Geometry check sheet. Reference: the model listing, model coordinates, mm. Round coordinates to 2 decimals unless told otherwise and drop trailing zeros. Order: outer loops, then holes, each group sorted by start corner. A loop starts at its lowest first (then second) coordinate and runs counter-clockwise, first axis right, second up.
(1) Go/stop test with flat-tipped pins: pin 1 (4 mm diameter, centred on y = 22.5, z = 2.5, fed in from +X); pin 2 (3 mm diameter, centred on x = 10.5, z = 5, fed in from -Y). Record where each tip stops, or that it passes through.
(2) Material ranges on line 1 along Y through (x, z) = (0, 2.95); line 2 along X through (y, z) = (15.5, 6); line 3 along Y through (x, z) = (8.5, 2), recorded low to high.
(3) Sectioned sample at A-A (x = 0). Record the boundary of the cut face in (y, z), plus the area to 3 significant figures.
(4) Release check for a two-part mould opening along Y. For faces 1 (the face through (-8.67, -39.05, 3.48)), 2 (the face through (-1, -8, 0)), 3 (the face through (5.97, 20.36, 3.47)) record: +Y half, -Y half, draft (parallel to the pull), parting line (faces both ways), or undercut.
(5) Sectioned sample at B-B (z = 3.75). Record the boundary of the cut face in (x, y), plus the area to 3 significant figures.
from build123d import *

# Parameters (mm, degrees)
F0_R     = 40
F0_R_2   = 11.1
F1_DEPTH = 7
F2_SIZE  = 2
F3_SIZE2 = 1.5
F3_SIZE  = 0.5


with BuildPart() as f1:
    # F0 (on Top) → F1 (new body)
    with BuildSketch(Plane.XY):
        Circle(F0_R)
        with Locations((0, 11)):
            Circle(F0_R_2, mode=Mode.SUBTRACT)
    extrude(amount=F1_DEPTH)

    # F2
    f2_edges = [f1.edges().sort_by_distance(p)[0] for p in [
        (-40, 0, 7),
        (-40, 0, 0),
    ]]
    chamfer(f2_edges, length=F2_SIZE)

    # F3
    f3_edges = [f1.edges().sort_by_distance(p)[0] for p in [
        (-11.1, 11, 0),
        (-11.1, 11, 7),
    ]]
    chamfer(f3_edges, length=F3_SIZE, length2=F3_SIZE2)


solid = f1.part
Answer below:
1. pin 1: stops at x = 34.35
1. pin 2: stops at y = -38.97
2. line 1: y = -40 to -0.1, 22.1 to 40
2. line 2: x = -35.79 to -10.33, 10.33 to 35.79
2. line 3: y = -39.09 to 3.86, 18.14 to 39.09
3. outline: (-40, 2) - (-38, 0) - (-0.6, 0) - (-0.1, 1.5) - (-0.1, 5.5) - (-0.6, 7) - (-38, 7) - (-40, 5) - close; (22.1, 1.5) - (22.6, 0) - (38, 0) - (40, 2) - (40, 5) - (38, 7) - (22.6, 7) - (22.1, 5.5) - close
3. area: 395 mm2
4. face 1: parting line
4. face 2: draft
4. face 3: undercut
5. outline: circle Ø80 at (0, 0); hole circle Ø22.2 at (0, 11)
5. area: 4,640 mm2
